```python
from build123d import *

# Parameters (mm, degrees)
SKETCH1_W           = 101.6
SKETCH1_H           = 25.4
BOSS_EXTRUDE1_DEPTH = 215.9
SKETCH3_R           = 5.207
CUT_EXTRUDE1_DEPTH  = 17.78
SKETCH4_R           = 5.08
BOSS_EXTRUDE3_DEPTH = 17.78


with BuildPart() as part:
    # Sketch1 → Boss-Extrude1 (new body)
    with BuildSketch(Plane(origin=(0, 0, 0), x_dir=(1, 0, 0), z_dir=(0, 1, 0))):
        with Locations((25.4, 12.7)):
            Rectangle(SKETCH1_W, SKETCH1_H)
    extrude(amount=BOSS_EXTRUDE1_DEPTH)

    # Sketch3 → Cut-Extrude1 (cut)
    with BuildSketch(Plane(origin=(0, 0, 0), x_dir=(-1, 0, 0), z_dir=(0, -1, 0))):
        with Locations(Location((5.08, 12.7, 0), (0, 0, 90))):
            Circle(SKETCH3_R)
        with Locations(Location((-55.88, 12.7, 0), (0, 0, 90))):
            Circle(SKETCH3_R)
    extrude(amount=-CUT_EXTRUDE1_DEPTH, mode=Mode.SUBTRACT)

    # Sketch4 → Boss-Extrude3 (add)
    with BuildSketch(Plane(origin=(0, 215.9, 0), x_dir=(1, 0, 0), z_dir=(0, 1, 0))):
        with Locations(Location((-5.08, 12.7, 0), (0, 0, 270))):
            Circle(SKETCH4_R)
        with Locations(Location((55.88, 12.7, 0), (0, 0, 270))):
            Circle(SKETCH4_R)
    extrude(amount=BOSS_EXTRUDE3_DEPTH)


solid = part.part
```
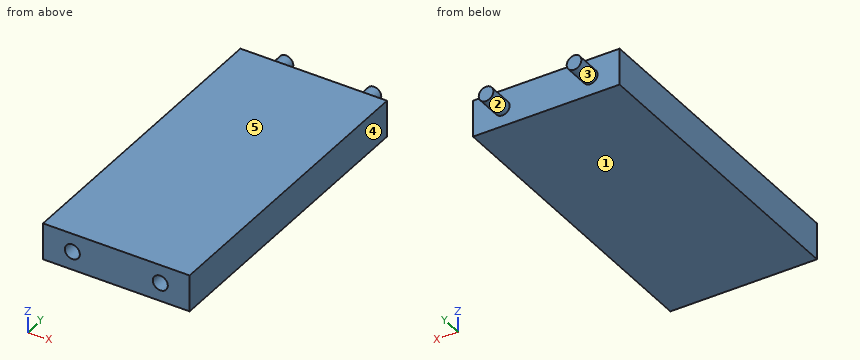
Here's how the part is built. I have some questions about the finished solid (model axes, mm). Face numbers are marked on the shaded views. A direction names the side the tool comes from. Give positions to 0.01 mm unless a question says otherwise; leave off trailing zeros. Order: outer loops, then holes, each group sorted by start corner. A loop starts at its lowest first (then second) coordinate and runs counter-clockwise, first axis right, second up. Notation, with made-up numbers: M -2,-16.75 L 23,-16.75 A12 ccw 23,-8.75 Z; hole C 77.5,17.25 d9. An arc over 180 degrees is marked long. Use a Markdown table: item, result. Add a question column.
1. Suppose I cut it at B-B (z = -12.7). List the corners of the cut face in (x, y) for me.
2. I need wall thicknesses on probe 1 along X at (y, z) = (14, -12.7); probe 2 along Z at (x, y) = (57, 11.5); probe 3 along Y at (x, z) = (15, -3.5). Which ranges of each line are inside material? Lowest first, please. Write a range as from..to.
3. Suppose I cut it at A-A (x = -5.08). List the corners of the cut face in (y, z) for me, and give its area (3 significant figures).
4. For pin 1 Ø3 at (x, z) = (44, -12) entering from +Y; pin 2 Ø3 at (x, z) = (54.5, -14.5) entering from -Y, each with a flat end and sliding along its axis, tell me the tip position at first contact or that it passes through.
5. Suppose I cut it at C-C (z = -22.75). List the corners of the cut face in (x, y) for me.
6. On a 3-axis mill with a long thin cutter (end or side, diameter ignored), from which of +Z, -Z, +X, -X, +Y, -Y can I reach the whole of each face in a straight line? I mean the marked faces 1 and 2. Say none if no direction works.
7. If we mould it in two halves opening along X, with no side actions, what happens to the marked faces 3, 4 and 5? For each: +X half, -X half, draft (parallel to the pull), parting line (faces both ways), or undercut.
Results list:
| question | item | result |
|---|---|---|
| 1 | outline | M -25.4,0 L -10.29,0 L -10.29,17.78 L 0.13,17.78 L 0.13,0 L 50.67,0 L 50.67,17.78 L 61.09,17.78 L 61.09,0 L 76.2,0 L 76.2,215.9 L 60.96,215.9 L 60.96,233.68 L 50.8,233.68 L 50.8,215.9 L 0,215.9 L 0,233.68 L -10.16,233.68 L -10.16,215.9 L -25.4,215.9 Z |
| 2 | probe 1 | x = -25.4..-10.29, 0.13..50.67, 61.09..76.2 |
| 2 | probe 2 | z = -25.4..-17.79, -7.61..0 |
| 2 | probe 3 | y = 0..215.9 |
| 3 | outline | M 0,-25.4 L 215.9,-25.4 L 215.9,-17.78 L 233.68,-17.78 L 233.68,-7.62 L 215.9,-7.62 L 215.9,0 L 0,0 L 0,-7.49 L 17.78,-7.49 L 17.78,-17.91 L 0,-17.91 Z |
| 3 | area | 5,480 mm² |
| 4 | pin 1 | stops at y = 215.9 |
| 4 | pin 2 | stops at y = 17.78 |
| 5 | outline | M -25.4,0 L 76.2,0 L 76.2,215.9 L -25.4,215.9 Z |
| 6 | face 1 | -Z, +X, -X, +Y, -Y |
| 6 | face 2 | +Y |
| 7 | face 3 | undercut |
| 7 | face 4 | +X half |
| 7 | face 5 | draft |
